Part model, mm, in its own coordinate system. Face numbers are marked on the shaded views. A direction names the side the tool comes from. Round coordinates to 2 decimals unless told otherwise and drop trailing zeros. Order: outer loops, then holes, each group sorted by start corner. A loop starts at its lowest first (then second) coordinate and runs counter-clockwise, first axis right, second up. Notation, with made-up numbers: M -2.75,8 L 31.25,8 A16 cw 31.25,34 Z; hole C -10,13 d10. An arc over 180 degrees is marked long. Write each question's results on one line, items separated by ' | '. Start each with the question number.
1. Probe L1, parallel to X at y = -9.5, z = 6; L2, parallel to Z at x = 0, y = -7.25; L3, parallel to Z at x = -65, y = -10.5. List the from-to ranges inside material, lowest first. Write a range as [from, to].
2. Band-saw the part on A-A, the plane x = 186.5. List the corners of the cut face in (y, z), then the cut area to 3 significant figures.
3. Drop flat-ended pins along their axis: pin 1 Ø4 at (x, z) = (-242.5, 27.5) entering from +Y; pin 2 Ø12.5 at (x, z) = (227.67, 81.4) entering from -Y; pin 3 Ø5 at (x, y) = (229, -6.5) entering from -Z; pin 4 Ø5 at (x, y) = (12.5, -11.5) entering from +Z. Give the stop position or say it passes through.
4. Which spindle directions (+Z, -Z, +X, -X, +Y, -Y) get a long thin tool onto all of the face, cutting with end or side? Do the marked faces 3 and 4. Say none if no direction does.
5. Two-plate mould, pull along Z, no slides. Class the marked faces 1 and 2: +Z half, -Z half, draft (parallel to the pull), parting line (faces both ways), or undercut.
```python
from build123d import *

# Parameters (mm, degrees)
SKETCH1_W                                    = 500
SKETCH1_H                                    = 16
BASE_EXTRUDE_DEPTH                           = 65
EXTRUSION_FOR_BLADE_CLAMPING_DEPTH           = 16
CUTAWAY_TO_BALANCE_BLADE_EXTRUSION_REACH     = 18
HOLES_FOR_WIRES_FROM_BLADES_REACH            = 18
MILLING_FOR_UPPERWIRE_PITCH_ADJUSTMENT_DEPTH = 5
SKETCH9_R                                    = 3.175
SLOTS_HOLE_FOR_UPPERWIRE_PITCH_ADJ_DEPTH     = 16
F_8_32_TAPPED_HOLE1_D                        = 3.4544
F_1_4_20_TAPPED_HOLE1_D                      = 5.1054
F_8_32_TAPPED_HOLE2_D                        = 3.4544
F_8_32_TAPPED_HOLE3_D                        = 3.4544
F_1_4_20_TAPPED_HOLE2_D                      = 5.1054
F_8_32_TAPPED_HOLE5_D                        = 3.4544
F_8_32_TAPPED_HOLE5_DEPTH                    = 12.2936
F_8_32_TAPPED_HOLE5_TIP                      = 1.037806461
F_8_32_TAPPED_HOLE6_D                        = 3.4544
F_8_32_TAPPED_HOLE6_DEPTH                    = 12.2936
F_8_32_TAPPED_HOLE6_TIP                      = 1.037806461
F_8_32_TAPPED_HOLE7_D                        = 3.4544
F_8_32_TAPPED_HOLE7_DEPTH                    = 12.2936
F_8_32_TAPPED_HOLE7_TIP                      = 1.037806461
F_8_32_TAPPED_HOLE8_D                        = 3.4544
F_8_32_TAPPED_HOLE8_DEPTH                    = 12.2936
F_8_32_TAPPED_HOLE8_TIP                      = 1.037806461
F_1_2_13_TAPPED_HOLE4_D                      = 10.71626


with BuildPart() as part:
    # Sketch1 → Base-Extrude (new body, symmetric)
    with BuildSketch(Plane.XY):
        with Locations((0, -8)):
            Rectangle(SKETCH1_W, SKETCH1_H)
    extrude(amount=BASE_EXTRUDE_DEPTH, both=True)

    # Sketch3 → Extrusion for Blade Clamping (add)
    with BuildSketch(Plane(origin=(0, 0, 0), x_dir=(-1, 0, 0), z_dir=(0, 1, 0))):
        Polygon((-210, 95), (-100, 65), (-250, 65), (-250, 95), align=None)
        Polygon((210, -95), (100, -65), (250, -65), (250, -95), align=None)
    extrude(amount=-EXTRUSION_FOR_BLADE_CLAMPING_DEPTH)

    # Sketch4 → Cutaway to Balance Blade Extrusion (cut, up to next)
    with BuildSketch(Plane(origin=(0, 0, 0), x_dir=(-1, 0, 0), z_dir=(0, 1, 0)), mode=Mode.PRIVATE) as cutaway_to_balance_blade_extrusion_sk1:
        Polygon((-205, -35), (-95, -65), (-250, -65), (-250, -35), align=None)
    cutaway_to_balance_blade_extrusion_tool1 = extrude(cutaway_to_balance_blade_extrusion_sk1.sketch, amount=-CUTAWAY_TO_BALANCE_BLADE_EXTRUSION_REACH, mode=Mode.PRIVATE) & part.part
    add(cutaway_to_balance_blade_extrusion_tool1.solids().sort_by_distance((194.958333, 0, -52.75))[0], mode=Mode.SUBTRACT)
    # Sketch4 → Cutaway to Balance Blade Extrusion (cut, up to next)
    with BuildSketch(Plane(origin=(0, 0, 0), x_dir=(-1, 0, 0), z_dir=(0, 1, 0)), mode=Mode.PRIVATE) as cutaway_to_balance_blade_extrusion_sk2:
        Polygon((250, 65), (250, 35), (205, 35), (95, 65), align=None)
    cutaway_to_balance_blade_extrusion_tool2 = extrude(cutaway_to_balance_blade_extrusion_sk2.sketch, amount=-CUTAWAY_TO_BALANCE_BLADE_EXTRUSION_REACH, mode=Mode.PRIVATE) & part.part
    add(cutaway_to_balance_blade_extrusion_tool2.solids().sort_by_distance((-194.958333, 0, 52.75))[0], mode=Mode.SUBTRACT)

    # Sketch5 → Holes for Wires from Blades (cut, up to next)
    with BuildSketch(Plane(origin=(0, 0, 0), x_dir=(-1, 0, 0), z_dir=(0, 1, 0)), mode=Mode.PRIVATE) as holes_for_wires_from_blades_sk1:
        with BuildLine():
            Line((-215, 8.5), (-215, -8.5))
            ThreePointArc((-215, -8.5), (-213.828427125, -11.328427125), (-211, -12.5))
            Line((-211, -12.5), (-179, -12.5))
            ThreePointArc((-179, -12.5), (-176.171572875, -11.328427125), (-175, -8.5))
            Line((-175, -8.5), (-175, 8.5))
            ThreePointArc((-175, 8.5), (-176.171572875, 11.328427125), (-179, 12.5))
            Line((-179, 12.5), (-211, 12.5))
            ThreePointArc((-211, 12.5), (-213.828427125, 11.328427125), (-215, 8.5))
        make_face()
    holes_for_wires_from_blades_tool1 = extrude(holes_for_wires_from_blades_sk1.sketch, amount=-HOLES_FOR_WIRES_FROM_BLADES_REACH, mode=Mode.PRIVATE) & part.part
    add(holes_for_wires_from_blades_tool1.solids().sort_by_distance((195, 0, 0))[0], mode=Mode.SUBTRACT)
    # Sketch5 → Holes for Wires from Blades (cut, up to next)
    with BuildSketch(Plane(origin=(0, 0, 0), x_dir=(-1, 0, 0), z_dir=(0, 1, 0)), mode=Mode.PRIVATE) as holes_for_wires_from_blades_sk2:
        with BuildLine():
            Line((211, 12.5), (179, 12.5))
            ThreePointArc((179, 12.5), (176.171572875, 11.328427125), (175, 8.5))
            Line((175, 8.5), (175, -8.5))
            ThreePointArc((175, -8.5), (176.171572875, -11.328427125), (179, -12.5))
            Line((179, -12.5), (211, -12.5))
            ThreePointArc((211, -12.5), (213.828427125, -11.328427125), (215, -8.5))
            Line((215, -8.5), (215, 8.5))
            ThreePointArc((215, 8.5), (213.828427125, 11.328427125), (211, 12.5))
        make_face()
    holes_for_wires_from_blades_tool2 = extrude(holes_for_wires_from_blades_sk2.sketch, amount=-HOLES_FOR_WIRES_FROM_BLADES_REACH, mode=Mode.PRIVATE) & part.part
    add(holes_for_wires_from_blades_tool2.solids().sort_by_distance((-195, 0, 0))[0], mode=Mode.SUBTRACT)

    # Sketch7 → Milling for UpperWire Pitch Adjustment (cut)
    with BuildSketch(Plane(origin=(0, 0, 0), x_dir=(-1, 0, 0), z_dir=(0, 1, 0))):
        with BuildLine():
            Line((-27, -7.83241743), (-27, 7.83241743))
            ThreePointArc((-27, 7.83241743), (-29.452904198, 14.39300772), (-35.60826899, 17.735098118))
            Line((-35.60826899, 17.735098118), (-86.60826899, 24.902680687))
            ThreePointArc((-86.60826899, 24.902680687), (-94.56059029, 22.547095802), (-98, 15))
            Line((-98, 15), (-98, -15))
            ThreePointArc((-98, -15), (-94.56059029, -22.547095802), (-86.60826899, -24.902680687))
            Line((-86.60826899, -24.902680687), (-35.60826899, -17.735098118))
            ThreePointArc((-35.60826899, -17.735098118), (-29.452904198, -14.39300772), (-27, -7.83241743))
        make_face()
        with BuildLine():
            Line((86.60826899, -24.902680687), (35.60826899, -17.735098118))
            ThreePointArc((35.60826899, -17.735098118), (29.452904198, -14.39300772), (27, -7.83241743))
            Line((27, -7.83241743), (27, 7.83241743))
            ThreePointArc((27, 7.83241743), (29.452904198, 14.39300772), (35.60826899, 17.735098118))
            Line((35.60826899, 17.735098118), (86.60826899, 24.902680687))
            ThreePointArc((86.60826899, 24.902680687), (94.56059029, 22.547095802), (98, 15))
            Line((98, 15), (98, -15))
            ThreePointArc((98, -15), (94.56059029, -22.547095802), (86.60826899, -24.902680687))
        make_face()
    extrude(amount=-MILLING_FOR_UPPERWIRE_PITCH_ADJUSTMENT_DEPTH, mode=Mode.SUBTRACT)

    # Sketch9 → Slots/Hole for UpperWire Pitch Adj (cut)
    with BuildSketch(Plane(origin=(0, 0, 0), x_dir=(-1, 0, 0), z_dir=(0, 1, 0))):
        with Locations((38, 0)):
            Circle(SKETCH9_R)
        with Locations((-38, 0)):
            Circle(SKETCH9_R)
        with BuildLine():
            ThreePointArc((-88.783028675, -15.654843384), (-86.289278515, -17.400986044), (-84.543135856, -14.907235885))
            ThreePointArc((-84.543135856, -14.907235885), (-85.011889491, -11.947641909), (-85.377069234, -8.973491571))
            ThreePointArc((-85.377069234, -8.973491571), (-87.742939989, -7.057647209), (-89.65878435, -9.423517964))
            ThreePointArc((-89.65878435, -9.423517964), (-89.275290607, -12.54682386), (-88.783028675, -15.654843384))
        make_face()
        with BuildLine():
            ThreePointArc((-84.543135856, 14.907235885), (-86.289278515, 17.400986044), (-88.783028675, 15.654843384))
            ThreePointArc((-88.783028675, 15.654843384), (-89.275290607, 12.54682386), (-89.65878435, 9.423517964))
            ThreePointArc((-89.65878435, 9.423517964), (-87.742939989, 7.057647209), (-85.377069234, 8.973491571))
            ThreePointArc((-85.377069234, 8.973491571), (-85.011889491, 11.947641909), (-84.543135856, 14.907235885))
        make_face()
        with BuildLine():
            ThreePointArc((88.783028675, 15.654843384), (89.275290607, 12.54682386), (89.65878435, 9.423517964))
            ThreePointArc((89.65878435, 9.423517964), (87.742939989, 7.057647209), (85.377069234, 8.973491571))
            ThreePointArc((85.377069234, 8.973491571), (85.011889491, 11.947641909), (84.543135856, 14.907235885))
            ThreePointArc((84.543135856, 14.907235885), (86.289278515, 17.400986044), (88.783028675, 15.654843384))
        make_face()
        with BuildLine():
            ThreePointArc((85.377069234, -8.973491571), (85.011889491, -11.947641909), (84.543135856, -14.907235885))
            ThreePointArc((84.543135856, -14.907235885), (86.289278515, -17.400986044), (88.783028675, -15.654843384))
            ThreePointArc((88.783028675, -15.654843384), (89.275290607, -12.54682386), (89.65878435, -9.423517964))
            ThreePointArc((89.65878435, -9.423517964), (87.742939989, -7.057647209), (85.377069234, -8.973491571))
        make_face()
    extrude(amount=-SLOTS_HOLE_FOR_UPPERWIRE_PITCH_ADJ_DEPTH, mode=Mode.SUBTRACT)

    # #8-32 Tapped Hole1 (through all)
    with Locations(Plane(origin=(0, 0, 6), x_dir=(1, 0, 0), z_dir=(0, 1, 0))):
        with Locations((0, 0), (0, 12)):
            Hole(F_8_32_TAPPED_HOLE1_D / 2)

    # 1/4-20 Tapped Hole1 (through all)
    with Locations(Plane(origin=(0, 0, 0), x_dir=(-1, 0, 0), z_dir=(0, 1, 0))):
        with Locations((-242.5, -27.5), (-242.5, 22.5), (242.5, 27.5), (242.5, -22.5)):
            Hole(F_1_4_20_TAPPED_HOLE1_D / 2)

    # #8-32 Tapped Hole2 (through all)
    with Locations(Plane(origin=(0, 0, 0), x_dir=(-1, 0, 0), z_dir=(0, 1, 0))):
        with Locations((-65, 45), (-85, 45), (85, 45), (65, 45), (85, -45), (65, -45), (-65, -45), (-85, -45)):
            Hole(F_8_32_TAPPED_HOLE2_D / 2)

    # #8-32 Tapped Hole3 (through all)
    with Locations(Plane.XZ.offset(16)):
        with Locations((-56, 26), (56, -26), (56, 26), (-56, -26)):
            Hole(F_8_32_TAPPED_HOLE3_D / 2)

    # 1/4-20 Tapped Hole2 (through all)
    with Locations(Plane(origin=(0, 0, 0), x_dir=(-1, 0, 0), z_dir=(0, 1, 0))):
        with Locations((0, 57.5), (0, -57.5)):
            Hole(F_1_4_20_TAPPED_HOLE2_D / 2)

    # #8-32 Tapped Hole5
    with Locations(Plane.XY.offset(59.7)):
        with Locations((-120, -8)):
            Hole(F_8_32_TAPPED_HOLE5_D / 2, depth=F_8_32_TAPPED_HOLE5_DEPTH)
            with Locations((0, 0, -(F_8_32_TAPPED_HOLE5_DEPTH + F_8_32_TAPPED_HOLE5_TIP / 2))):  # 118° drill point
                Cone(0, F_8_32_TAPPED_HOLE5_D / 2, F_8_32_TAPPED_HOLE5_TIP, mode=Mode.SUBTRACT)

    # #8-32 Tapped Hole6
    with Locations(Plane.XY.offset(71)):
        with Locations((120, -8)):
            Hole(F_8_32_TAPPED_HOLE6_D / 2, depth=F_8_32_TAPPED_HOLE6_DEPTH)
            with Locations((0, 0, -(F_8_32_TAPPED_HOLE6_DEPTH + F_8_32_TAPPED_HOLE6_TIP / 2))):  # 118° drill point
                Cone(0, F_8_32_TAPPED_HOLE6_D / 2, F_8_32_TAPPED_HOLE6_TIP, mode=Mode.SUBTRACT)

    # #8-32 Tapped Hole7
    with Locations(Plane(origin=(0, 0, -59.7), x_dir=(-1, 0, 0), z_dir=(0, 0, -1))):
        with Locations((-120, -8)):
            Hole(F_8_32_TAPPED_HOLE7_D / 2, depth=F_8_32_TAPPED_HOLE7_DEPTH)
            with Locations((0, 0, -(F_8_32_TAPPED_HOLE7_DEPTH + F_8_32_TAPPED_HOLE7_TIP / 2))):  # 118° drill point
                Cone(0, F_8_32_TAPPED_HOLE7_D / 2, F_8_32_TAPPED_HOLE7_TIP, mode=Mode.SUBTRACT)

    # #8-32 Tapped Hole8
    with Locations(Plane(origin=(0, 0, -71), x_dir=(-1, 0, 0), z_dir=(0, 0, -1))):
        with Locations((120, -8)):
            Hole(F_8_32_TAPPED_HOLE8_D / 2, depth=F_8_32_TAPPED_HOLE8_DEPTH)
            with Locations((0, 0, -(F_8_32_TAPPED_HOLE8_DEPTH + F_8_32_TAPPED_HOLE8_TIP / 2))):  # 118° drill point
                Cone(0, F_8_32_TAPPED_HOLE8_D / 2, F_8_32_TAPPED_HOLE8_TIP, mode=Mode.SUBTRACT)

    # 1/2-13 Tapped Hole4 (through all)
    with Locations(Plane(origin=(-232.778633851, 0, -47.189591945), x_dir=(0, 0, 1), z_dir=(0, 1, 0))):
        with Locations((0, 0), (-34.215003793, 5.113466578), (94.37918389, 465.557267702), (128.594187683, 460.443801124)):
            Hole(F_1_2_13_TAPPED_HOLE4_D / 2)


solid = part.part
```
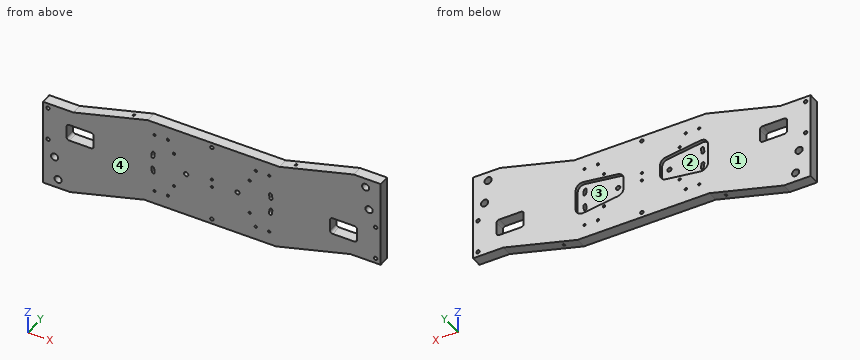
Solution:
1) L1: [-250, -215], [-175, -1.73], [1.73, 175], [215, 250] | L2: [-65, -60.05], [-54.95, -7.73], [-4.27, 4.27], [7.73, 54.95], [60.05, 65] | L3: [-65, -46.73], [-43.27, 43.27], [46.73, 65]
2) outline: M -16,-40.05 L 0,-40.05 L 0,-12.5 L -16,-12.5 Z; M -16,12.5 L 0,12.5 L 0,88.59 L -16,88.59 Z | area: 1,660 mm^2
3) pin 1: through | pin 2: y = -16 | pin 3: z = -35 | pin 4: z = 65
4) face 3: +Y | face 4: +Z, -Z, +X, -X, -Y
5) face 1: draft | face 2: undercut
